Geometry check sheet. Reference: the model listing, model coordinates, mm. Face numbers are marked on the shaded views. A direction names the side the tool comes from. Round coordinates to 2 decimals unless told otherwise and drop trailing zeros. Loops run counter-clockwise (first coordinate to the right, second up) from the corner with the lowest first, then second, coordinate; pieces in that order, holes last. Notation, with made-up numbers: (58, 81.5) -> (88, 81.5) arc R23 cw to (88, 99.5) -> close; hole circle Ø9 at (-36.75, 12.5). An arc over 180 degrees is marked (long way). Use one line per item in the form item = value.
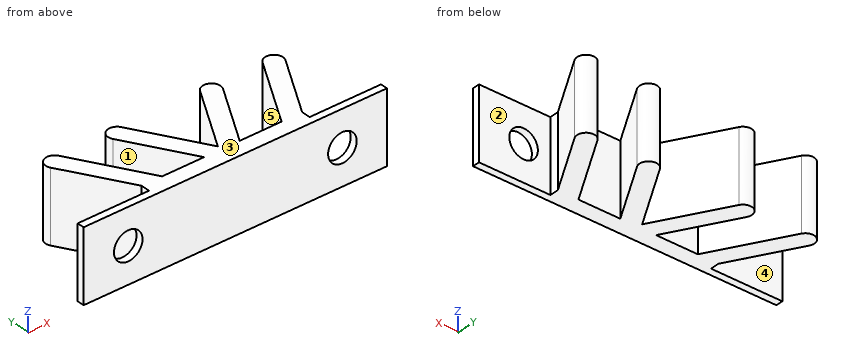
Autodesk Inventor part; units mm, degrees
ref_plane "YZ Plane" through (0, 0, 0) normal (1, 0, 0) x (0, 1, 0)
ref_plane "XZ Plane" through (0, 0, 0) normal (0, 1, 0) x (-1, 0, 0)
ref_plane "XY Plane" through (0, 0, 0) normal (0, 0, 1) x (1, 0, 0)
sketch "Skizze1" plane through (0, 0, 0) normal (0, 0, 1) x (1, 0, 0)
  line L0 (-17, 0) -> (17, 0)
  line L1 (0, 2.16) -> (0, -0.36)
  line L2 (-17, 0) -> (-17, 0.8)
  line L3 (17, 0.8) -> (17, 0)
  line L4 (-17, 0.8) -> (-9, 0.8)
  line L5 (-9, 0.8) -> (-9, 1.8)
  line L6 (-9, 1.8) -> (9, 1.8)
  line L7 (9, 1.8) -> (9, 0.8)
  line L8 (9, 0.8) -> (17, 0.8)
  point P0 (0, 0)
  dimension "d2" = 0.8
  dimension "d3" = 34
  dimension "d28" = 1
  dimension "d29" = 18
extrude "Extrusion1" add sketch "Skizze1" along normal blind 8
sketch "Skizze2" plane through (0, 0, 0) normal (0, 0, 1) x (1, 0, 0)
  line L0 (-17, 0) -> (17, 0) construction
  line L1 (17, 0) -> (17, 0.8) construction
  line L2 (-9, 0.8) -> (-17, 0.8) construction
  line L3 (-17, 0.8) -> (-17, 0) construction
  line L4 (-9, 1.8) -> (-13.1569, 9)
  line L5 (-6.6906, 1.8) -> (-9, 1.8)
  line L6 (-6.6906, 1.8) -> (-11.4249, 10)
  arc A0 (-11.4249, 10) -> (-13.1569, 9) centre (-12.2909, 9.5) ccw
  line L7 (-17, 0.8) -> (-17, 0.8) construction
  line L8 (-17, 0.8) -> (-17, 10.5) construction
  line L9 (-17, 10.5) -> (17, 10.5) construction
  line L10 (17, 10.5) -> (17, 0.8) construction
  line L11 (17, 0.8) -> (-9, 0.8) construction
  line L12 (0, 13.8837) -> (0, -2.3139) construction
  arc A1 (-10.865, 10.5) -> (-17, 0.8) centre (-7.8453, 1.8) ccw construction
  line L13 (17, 0.8) -> (9, 0.8)
  line L14 (9, 0.8) -> (9, 1.8)
  line L15 (9, 1.8) -> (-9, 1.8) construction
  line L16 (-9, 1.8) -> (-9, 0.8)
  point P0 (0, 0)
  dimension "d10" = 2
  dimension "d11" = 60
  dimension "d12" = 34
  dimension "d14" = 10.5
extrude "Extrusion2" add sketch "Skizze2" along normal blind 8
pattern_linear "Rechteckige Anordnung1" count 2 spacing 7 along (1, 0, 0) of "Extrusion2"
mirror "Spiegeln1" about plane through (0, 0, 0) normal (1, 0, 0) of "Extrusion2", "Rechteckige Anordnung1"
sketch "Skizze3" plane through (-17, 0, 0) normal (0, -1, 0) x (1, 0, 0)
  line L0 (17, 9.6) -> (17, -1.6)
  line L1 (0, 0) -> (34, 0)
  line L2 (34, 0) -> (34, 8)
  line L3 (0, 8) -> (34, 8)
  line L4 (0, 0) -> (0, 8)
  line L5 (0, 0) -> (0, 8) construction
  line L6 (0, 4) -> (34, 4) construction
  point P0 (17, 0)
  point P1 (5, 4)
  point P2 (29, 4)
  dimension "d20" = 24
hole "Bohrung1" at (-12, 0, 4) at (12, 0, 4) direction (0, 1, 0) diameter 3.2 depth 2 tip angle 118
properties part number "Dribblerdaempfer V2" material "Gummi, Silikon"
1. Tool access check on the marked faces 1, 2, 3, 4 and 5. Record the directions out of +Z, -Z, +X, -X, +Y, -Y that give a thin tool (end or side, any length) a straight path to the whole face; none if there is none.
Return value:
face_1 = +Z, -Z
face_2 = +Z, -Z, +X
face_3 = +Z, +X, -X, +Y, -Y
face_4 = +Z, -Z, -X
face_5 = +Z, -Z, +Y
2. Section check A-A (z = 4). Count the separate pieces of the cut face and the enclosed holes in it, then the cut area to 3 significant figures.
Return value:
separate_pieces = 3
enclosed_holes = 0
area = 117 mm2
3. Material ranges on line 1 along X through (y, z) = (0.45, 4); line 2 along X through (y, z) = (10, 5.5); line 3 along Z through (x, y) = (12, 0.65), recorded low to high.
Return value:
line_1 = -17 to -13.6, -10.4 to 10.4, 13.6 to 17
line_2 = -13.16 to -11.42, -6.16 to -4.42, 4.42 to 6.16, 11.42 to 13.16
line_3 = 0 to 2.4, 5.6 to 8
4. Section check C-C (y = 9.5). Record the boundary of the cut face in (x, z), then the cut area to 3 significant figures.
Return value:
outline = (-13.29, 0) -> (-11.14, 0) -> (-11.14, 8) -> (-13.29, 8) -> close; (-6.29, 0) -> (-4.14, 0) -> (-4.14, 8) -> (-6.29, 8) -> close; (4.14, 0) -> (6.29, 0) -> (6.29, 8) -> (4.14, 8) -> close; (11.14, 0) -> (13.29, 0) -> (13.29, 8) -> (11.14, 8) -> close
area = 68.9 mm2
5. Gauge pin test, flat ends, axial feed: pin 1 (1 mm diameter, centred on y = 1.5, z = 1, fed in from +X); pin 2 (1.4 mm diameter, centred on x = 4.5, z = 5.5, fed in from +Y); pin 3 (2 mm diameter, centred on y = 6.5, z = 1.5, fed in from +X). Record the tip position at first contact, or that the pin passes through.
Return value:
pin_1 = 9.12
pin_2 = 10.5
pin_3 = 12.29
6. Section check B-B (x = 12). Record the boundary of the cut face in (y, z), then the cut area to 3 significant figures.
Return value:
outline = (0, 0) -> (0.8, 0) -> (0.8, 2.4) -> (0, 2.4) -> close; (0, 5.6) -> (0.8, 5.6) -> (0.8, 8) -> (0, 8) -> close; (7, 0) -> (10.46, 0) -> (10.46, 8) -> (7, 8) -> close
area = 31.5 mm2
7. Section check D-D (x = -5.5). Record the boundary of the cut face in (y, z), then the cut area to 3 significant figures.
Return value:
outline = (0, 0) -> (1.8, 0) -> (1.8, 8) -> (0, 8) -> close; (7.86, 0) -> (10.48, 0) -> (10.48, 8) -> (7.86, 8) -> close
area = 35.3 mm2
